The model under review builds one solid part; all positions refer to its coordinate system, in mm. A direction names the side the tool comes from. Round coordinates to 2 decimals unless told otherwise and drop trailing zeros. Write each loop counter-clockwise with the first axis right and the second up, starting at its lowest first coordinate (ties: lowest second). Pieces come first, ordered by that corner, then holes. Notation, with made-up numbers: (78.5, 13) -> (127.5, 13) arc R26 cw to (127.5, 52) -> close; hole circle Ø9 at (0.5, -7). An arc over 180 degrees is marked (long way). Return JSON: item names as keys, results as strings. Group by question number.
1. Take a section at C-C, the plane z = 0. Give the number of separate pieces and of enclosed holes in the cut face, then the cut area to 3 significant figures.
2. Mouldability with a two-part tool opening along X and no side actions: class faces 1 (the flat face through (2, 6, -23)), 2 (the flat face through (1, 0, 10)), 3 (the cylindrical face through (1.689, 1.521, 39.964)) as pulls with the +X half, pulls with the -X half, needs draft (parallel to the pull), parting line crosses it, or undercut.
3. Take a section at D-D, the plane x = 34. Write out the cut boundary in (y, z).
4. Tool access review of faces 4 (the flat face through (9.7, 7, 1.4)), 5 (the cylindrical face through (15.755, 8.874, 6.385)), 6 (the flat face through (2.901, 4, -26)), 7 (the flat face through (-1, 18, -8)): name each direction out of +Z, -Z, +X, -X, +Y, -Y from which nothing blocks a thin tool from reaching the whole face with its end or side.
5. For line 1 along Z through (x, y) = (0, 2.2); line 2 along Z through (x, y) = (15, 15.25); line 3 along Z through (x, y) = (2, 3.25), list the stretches that pass through material, from the lowest coordinate up. Write a range as from..to.
6. Take a section at A-A, the plane x = 25.5. Write out the cut boundary in (y, z).
7. Take a section at B-B, the plane z = 23. Write out the cut boundary in (x, y), then the cut area to 3 significant figures.
8. Clearance check with flat-ended pins moving along their axes: P1, Ø2.5, axis at x = -16, z = -13, coming from the -Y side; P2, Ø4.5, axis at x = 11.5, y = 1, coming from the +Z side; P3, Ø5.5, axis at x = 11.5, z = 0.5, coming from the -Y side; P4, Ø1.5, axis at y = 3.5, z = 8, coming from the +X side. State where each tip first meets the part, or that it passes through.
from build123d import *

# Parameters (mm, degrees)
CORTAR_EXTRUIR1_DEPTH      = 13
CROQUIS3_R                 = 1.7
CORTAR_EXTRUIR2_DEPTH      = 17
CORTAR_EXTRUIR3_DEPTH      = 1.5
CORTAR_EXTRUIR3_DEPTH_BACK = 1.5
CROQUIS5_R                 = 5
CORTAR_EXTRUIR4_DEPTH      = 18
CROQUIS6_R                 = 8.2
CORTAR_EXTRUIR5_DEPTH      = 9
CROQUIS7_W                 = 30.6
CROQUIS7_H                 = 7
CORTAR_EXTRUIR6_DEPTH      = 4
CROQUIS8_R                 = 1.7
CORTAR_EXTRUIR7_DEPTH      = 14
CORTAR_EXTRUIR8_DEPTH      = 11
CORTAR_EXTRUIR9_DEPTH      = 18
CROQUIS11_R                = 1.7
CORTAR_EXTRUIR10_DEPTH     = 18
CROQUIS12_R                = 2.95
CORTAR_EXTRUIR11_DEPTH     = 3


with BuildPart() as part:
    # Croquis1 → Revolución1 (revolve)
    with BuildSketch(Plane.XY):
        Polygon((0, 0), (40, 0), (40, 3), (37, 3), (37, 18), (0, 18), align=None)
    revolve(axis=Axis((0, 18, 0), (0, -1, 0)))

    # Croquis2 → Cortar-Extruir1 (cut)
    with BuildSketch(Plane.XZ):
        Polygon((-11.5, -19.5), (11.5, -19.5), (11.5, -23), (5, -29.5), (5, -54.5), (2.5, -54.5), (2.5, -29.5), (9, -23), (-9, -23), (-2.5, -29.5), (-2.5, -54.5), (-5, -54.5), (-5, -29.5), (-11.5, -23), align=None)
    extrude(amount=-CORTAR_EXTRUIR1_DEPTH, mode=Mode.SUBTRACT)

    # Croquis3 → Cortar-Extruir2 (cut)
    with BuildSketch(Plane.XY.offset(-40)):
        with Locations((0, 6.5)):
            Circle(CROQUIS3_R)
    extrude(amount=CORTAR_EXTRUIR2_DEPTH, mode=Mode.SUBTRACT)

    # Croquis4 → Cortar-Extruir3 (cut, two sides)
    with BuildSketch(Plane.XY.offset(-25.85)) as cortar_extruir3_sk:
        Polygon((0, 9.85), (-2.901185103, 8.175), (-2.901185103, 4.825), (-2.901185103, -1.825), (2.901185103, -1.825), (2.901185103, 4.825), (2.901185103, 8.175), align=None)
    extrude(amount=CORTAR_EXTRUIR3_DEPTH, mode=Mode.SUBTRACT)
    extrude(cortar_extruir3_sk.sketch, amount=-CORTAR_EXTRUIR3_DEPTH_BACK, mode=Mode.SUBTRACT)

    # Croquis5 → Cortar-Extruir4 (cut)
    with BuildSketch(Plane(origin=(0, 18, 0), x_dir=(1, 0, 0), z_dir=(0, 1, 0))):
        Circle(CROQUIS5_R)
    extrude(amount=-CORTAR_EXTRUIR4_DEPTH, mode=Mode.SUBTRACT)

    # Croquis6 → Cortar-Extruir5 (cut)
    with BuildSketch(Plane.XZ):
        Circle(CROQUIS6_R)
    extrude(amount=-CORTAR_EXTRUIR5_DEPTH, mode=Mode.SUBTRACT)

    # Croquis7 → Cortar-Extruir6 (cut)
    with BuildSketch(Plane.XZ):
        Rectangle(CROQUIS7_W, CROQUIS7_H)
    extrude(amount=-CORTAR_EXTRUIR6_DEPTH, mode=Mode.SUBTRACT)

    # Croquis8 → Cortar-Extruir7 (cut)
    with BuildSketch(Plane.XZ.offset(-4)):
        with Locations((-11, 0)):
            Circle(CROQUIS8_R)
        with Locations((11, 0)):
            Circle(CROQUIS8_R)
    extrude(amount=-CORTAR_EXTRUIR7_DEPTH, mode=Mode.SUBTRACT)

    # Croquis9 → Cortar-Extruir8 (cut)
    with BuildSketch(Plane(origin=(0, 18, 0), x_dir=(1, 0, 0), z_dir=(0, 1, 0))):
        Polygon((-11, 3.35), (-13.901185103, 1.675), (-13.901185103, -1.675), (-11, -3.35), (-8.098814897, -1.675), (-8.098814897, 1.675), align=None)
        Polygon((11, 3.35), (8.098814897, 1.675), (8.098814897, -1.675), (11, -3.35), (13.901185103, -1.675), (13.901185103, 1.675), align=None)
    extrude(amount=-CORTAR_EXTRUIR8_DEPTH, mode=Mode.SUBTRACT)

    # Croquis10 → Cortar-Extruir9 (cut)
    with BuildSketch(Plane.XZ):
        with BuildLine():
            Line((9.447221814, 16.363068172), (14.966629547, 25.922962794))
            ThreePointArc((14.966629547, 25.922962794), (16.245761141, 26.871003909), (17.811925712, 26.584493647))
            ThreePointArc((17.811925712, 26.584493647), (29.56414504, 12.245869836), (31.393009189, -6.203142275))
            ThreePointArc((31.393009189, -6.203142275), (30.48815695, -7.513181213), (28.913308024, -7.747297536))
            Line((28.913308024, -7.747297536), (18.250631073, -4.890241857))
            ThreePointArc((18.250631073, -4.890241857), (17.091330505, -4.048287785), (16.792661883, -2.64698071))
            ThreePointArc((16.792661883, -2.64698071), (15.705952053, 6.50561835), (10.002507082, 13.745903101))
            ThreePointArc((10.002507082, 13.745903101), (9.222823954, 14.947967445), (9.447221814, 16.363068172))
        make_face()
    cortar_extruir9 = extrude(amount=-CORTAR_EXTRUIR9_DEPTH, mode=Mode.SUBTRACT)

    # Simetría1: Cortar-Extruir9 across plane
    add(cortar_extruir9.mirror(Plane(origin=(0, 0, 0), x_dir=(0, 0, 1), z_dir=(1, 0, 0))), mode=Mode.SUBTRACT)

    # Croquis11 → Cortar-Extruir10 (cut)
    with BuildSketch(Plane.XZ):
        with Locations((-16, -13)):
            Circle(CROQUIS11_R)
        with Locations((16, -13)):
            Circle(CROQUIS11_R)
        with Locations((0, 18)):
            Circle(CROQUIS11_R)
    extrude(amount=-CORTAR_EXTRUIR10_DEPTH, mode=Mode.SUBTRACT)

    # Croquis12 → Cortar-Extruir11 (cut)
    with BuildSketch(Plane.XZ):
        with Locations((-16, -13)):
            Circle(CROQUIS12_R)
        with Locations((16, -13)):
            Circle(CROQUIS12_R)
        with Locations((0, 18)):
            Circle(CROQUIS12_R)
    extrude(amount=-CORTAR_EXTRUIR11_DEPTH, mode=Mode.SUBTRACT)


solid = part.part
Output:
{
 "1": {"separate pieces": "8", "enclosed holes": "0", "area": "368 mm^2"},
 "2": {"face 1": "undercut", "face 2": "needs draft", "face 3": "parting line crosses it"},
 "3": {"outline": "(0, -21.07) -> (3, -21.07) -> (3, -14.59) -> (18, -14.59) -> (18, 14.59) -> (3, 14.59) -> (3, 21.07) -> (0, 21.07) -> close"},
 "4": {"face 4": "+Y", "face 5": "+Y, -Y", "face 6": "-Y", "face 7": "+Z, -Z, +X, -X, +Y"},
 "5": {"line 1": "z = -40..-27.35, -24.35..-23, -19.5..-8.2, 8.2..15.05, 20.95..40", "line 2": "z = -33.82..-14.37, -11.63..8, 25.98..33.82", "line 3": "z = -36.95..-27.35, -24.35..-23, -19.5..-7.95, 7.95..36.95"},
 "6": {"outline": "(0, -30.82) -> (3, -30.82) -> (3, -26.81) -> (18, -26.81) -> (18, -6.83) -> (0, -6.83) -> close; (0, 19.33) -> (18, 19.33) -> (18, 26.81) -> (3, 26.81) -> (3, 30.82) -> (0, 30.82) -> close"},
 "7": {"outline": "(-32.73, 0) -> (-22.25, 0) -> (-22.25, 18) -> (-28.98, 18) -> (-28.98, 3) -> (-32.73, 3) -> close; (-13.28, 0) -> (13.28, 0) -> (13.28, 18) -> (-13.28, 18) -> close; (22.25, 0) -> (32.73, 0) -> (32.73, 3) -> (28.98, 3) -> (28.98, 18) -> (22.25, 18) -> close", "area": "743 mm^2"},
 "8": {"P1": "passes through", "P2": "stops at z = 38.92", "P3": "stops at y = 4", "P4": "stops at x = 39.3"}
}
